Design review of the part built by this model. Coordinates are the model's own, in mm. Face numbers are marked on the shaded views. A direction names the side the tool comes from. Round coordinates to 2 decimals unless told otherwise and drop trailing zeros. Order: outer loops, then holes, each group sorted by start corner. A loop starts at its lowest first (then second) coordinate and runs counter-clockwise, first axis right, second up.
from build123d import *

# Parameters (mm, degrees)
BOSS_EXTRU_1_DEPTH      = 44
ESQUISSE3_R             = 1.5
ENL_V_MAT_EXTRU_2_DEPTH = 16.1
ESQUISSE4_R             = 4
ENL_V_MAT_EXTRU_3_DEPTH = 2
ESQUISSE5_W             = 6
ESQUISSE5_H             = 4
ENL_V_MAT_EXTRU_4_DEPTH = 45


with BuildPart() as part:
    # Esquisse1 → Boss.-Extru.1 (new body)
    with BuildSketch(Plane.XY):
        Polygon((0, 15.1), (17.7, 15.1), (17.7, 10.1), (14.15, 10.1), (14.15, 9.1), (11.35, 9.1), (11.35, 10.1), (7.7, 10.1), (7.7, 6.45), (8.7, 6.45), (8.7, 3.65), (7.7, 3.65), (7.7, 0), (0, 0), align=None)
    extrude(amount=BOSS_EXTRU_1_DEPTH)

    # Esquisse3 → Enlèv. mat.-Extru.2 (cut, through all)
    with BuildSketch(Plane(origin=(0, 15.1, 0), x_dir=(1, 0, 0), z_dir=(0, 1, 0))):
        with Locations((12.7, -22)):
            Circle(ESQUISSE3_R)
    extrude(amount=-ENL_V_MAT_EXTRU_2_DEPTH, mode=Mode.SUBTRACT)

    # Esquisse4 → Enlèv. mat.-Extru.3 (cut)
    with BuildSketch(Plane(origin=(0, 15.1, 0), x_dir=(1, 0, 0), z_dir=(0, 1, 0))):
        with Locations((12.7, -22)):
            Circle(ESQUISSE4_R)
    extrude(amount=-ENL_V_MAT_EXTRU_3_DEPTH, mode=Mode.SUBTRACT)

    # Symétrie1: part across plane


with BuildPart() as part_1:
    add(part.part)
    add(part.part.mirror(Plane(origin=(0, 0, 44), x_dir=(0, 0, 1), z_dir=(1, 0, 0))))

    # Esquisse5 → Enlèv. mat.-Extru.4 (cut, through all)
    with BuildSketch(Plane.XY.offset(44)):
        with Locations((0, 7.1)):
            Rectangle(ESQUISSE5_W, ESQUISSE5_H)
    extrude(amount=-ENL_V_MAT_EXTRU_4_DEPTH, mode=Mode.SUBTRACT)


solid = part_1.part
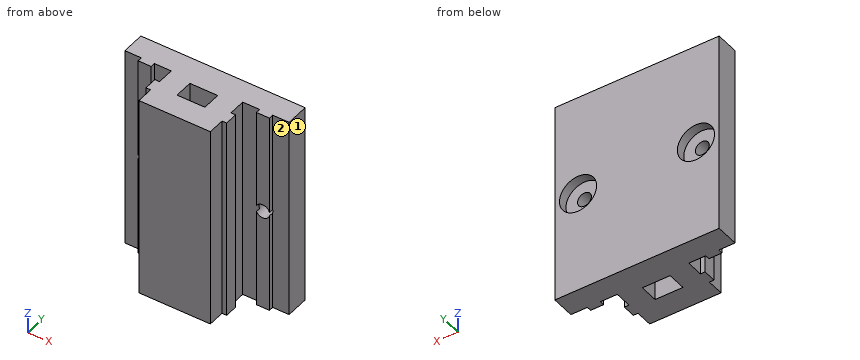
1) Clearance check with flat-ended pins moving along their axes: P1, Ø2, axis at y = 5.5, z = 20, coming from the -X side; P2, Ø2, axis at y = 9, z = 39, coming from the -X side; P3, Ø4.5, axis at y = 7.5, z = 17.5, coming from the +X side. State where each tip first meets the part, or that it passes through.
Results:
P1: stops at x = -8.7
P2: stops at x = -14.15
P3: stops at x = 14.15
2) Take a section at A-A on x = 12.7. Give the boundary of the cut face in (y, z), plus the area to 3 significant figures.
Results:
outline: (9.1, 0) - (15.1, 0) - (15.1, 18) - (13.1, 18) - (13.1, 20.5) - (9.1, 20.5) - close; (9.1, 23.5) - (13.1, 23.5) - (13.1, 26) - (15.1, 26) - (15.1, 44) - (9.1, 44) - close
area: 236 mm2
3) Take a section at C-C on y = 7. Give the boundary of the cut face in (x, z), plus the area to 3 significant figures.
Results:
outline: (-7.7, 0) - (-3, 0) - (-3, 44) - (-7.7, 44) - close; (3, 0) - (7.7, 0) - (7.7, 44) - (3, 44) - close
area: 414 mm2
4) Take a section at B-B on z = 5. Give the boundary of the cut face in (x, y), plus the area to 3 significant figures.
Results:
outline: (-17.7, 10.1) - (-14.15, 10.1) - (-14.15, 9.1) - (-11.35, 9.1) - (-11.35, 10.1) - (-7.7, 10.1) - (-7.7, 6.45) - (-8.7, 6.45) - (-8.7, 3.65) - (-7.7, 3.65) - (-7.7, 0) - (7.7, 0) - (7.7, 3.65) - (8.7, 3.65) - (8.7, 6.45) - (7.7, 6.45) - (7.7, 10.1) - (11.35, 10.1) - (11.35, 9.1) - (14.15, 9.1) - (14.15, 10.1) - (17.7, 10.1) - (17.7, 15.1) - (-17.7, 15.1) - close; hole (-3, 5.1) - (3, 5.1) - (3, 9.1) - (-3, 9.1) - close
area: 320 mm2
5) For the marked faces 1 and 2, list the 3-axis set-ups (+Z, -Z, +X, -X, +Y, -Y) from which the entire face can be reached by the end or side of a thin tool; tool diameter is ignored.
Results:
face 1: +Z, -Z, +X, +Y, -Y
face 2: +Z, -Z, +X, -Y
6) To check wall thickness, follow line 1 along X through (y, z) = (13.75, 22); line 2 along Z through (x, y) = (-12.7, 14.6); line 3 along X through (y, z) = (6.25, 29). State the ranges of each line that lie inside material, in increasing order.
Results:
line 1: x = -17.7 to -16.7, -8.7 to 8.7, 16.7 to 17.7
line 2: z = 0 to 18, 26 to 44
line 3: x = -8.7 to -3, 3 to 8.7
